The listing builds one solid part. Answer for the finished solid, in the listing's coordinates (mm). Face numbers are marked on the shaded views. A direction names the side the tool comes from. Round coordinates to 2 decimals unless told otherwise and drop trailing zeros. Write each loop counter-clockwise with the first axis right and the second up, starting at its lowest first coordinate (ties: lowest second). Pieces come first, ordered by that corner, then holes. Notation, with made-up numbers: M 42.5,87 L 99.5,87 A6 cw 99.5,92 Z; hole C 23,58.25 d10. An arc over 180 degrees is marked long. One line per item, written item: value. Start each with the question number.
(1) Consider probe 1 along X at (y, z) = (0, 6.5); probe 2 along X at (y, z) = (6, 10); probe 3 along Y at (x, z) = (0, 2.5). Determine where each line is inside the solid, lowest interval first.
(2) Section C-C (z = 5) is taken. Determine the outline of the cut face in (x, y).
(3) Section B-B (x = 0) is taken. Determine the outline of the cut face in (y, z).
(4) Given P1, Ø3, axis at x = 2, y = -16.5, coming from the +Z side; P2, Ø23, axis at x = 0, y = 0, coming from the +Z side, each flat-ended and moving along its own axis, determine where each tip first touches the part or whether it passes through.
(5) Section D-D (y = -15) is taken. Determine the outline of the cut face in (x, z), plus the area to 3 significant figures.
(6) Section A-A (y = 0) is taken. Determine the outline of the cut face in (x, z), plus the area to 3 significant figures.
(7) For a pull along X with two mould halves and no side action, classify the marked faces 1, 2, 3 and 4 as released by +X, released by -X, zero draft, split by the parting line, or undercut.
(8) For the marked faces 5, 6 and 7, determine the directions among +Z, -Z, +X, -X, +Y, -Y from which every point of the face is accessible in a straight line to the end or side of a thin tool.
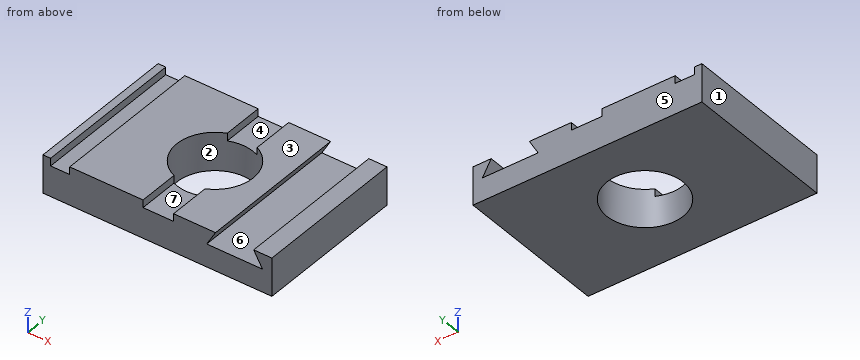
```python
from build123d import *

# Parameters (mm, degrees)
F0_W     = 76.2
F0_H     = 50.8
F0_R     = 12.7
F1_DEPTH = 12.7
F2_W     = 6.35
F2_H     = 50.8
F3_DEPTH = 2.54
F5_DEPTH = 50.801


with BuildPart() as f1:
    # F0 (on Top) → F1 (new body)
    with BuildSketch(Plane.XY):
        Rectangle(F0_W, F0_H)
        Circle(F0_R, mode=Mode.SUBTRACT)
    extrude(amount=F1_DEPTH)

    # F2 (on face) → F3 (cut)
    with BuildSketch(Plane.XY.offset(12.7)):
        with Locations((-32.385, 0)):
            Rectangle(F2_W, F2_H)
        with BuildLine():
            Line((5.37053629, 25.4), (-4.78946371, 25.4))
            Line((-4.78946371, 25.4), (-4.78946371, 11.7622717776))
            ThreePointArc((-4.78946371, 11.7622717776), (0.3170199067, 12.6960426267), (5.37053629, 11.5085767999))
            Line((5.37053629, 11.5085767999), (5.37053629, 25.4))
        make_face()
        with BuildLine():
            Line((-4.78946371, -11.7622717776), (-4.78946371, -25.4))
            Line((-4.78946371, -25.4), (5.37053629, -25.4))
            Line((5.37053629, -25.4), (5.37053629, -11.5085767999))
            ThreePointArc((5.37053629, -11.5085767999), (0.3170199067, -12.6960426267), (-4.78946371, -11.7622717776))
        make_face()
    extrude(amount=-F3_DEPTH, mode=Mode.SUBTRACT)

    # F4 (on face) → F5 (cut, through all)
    with BuildSketch(Plane.XZ.offset(25.4)):
        Polygon((32.04053629, 12.7), (19.34053629, 12.7), (16.4075969225, 7.62), (34.9734756574, 7.62), align=None)
    extrude(amount=-F5_DEPTH, mode=Mode.SUBTRACT)


solid = f1.part
```
Recorded:
1. probe 1: x = -38.1 to -12.7, 12.7 to 38.1
1. probe 2: x = -38.1 to -11.19, 11.19 to 17.78, 33.6 to 38.1
1. probe 3: y = -25.4 to -12.7, 12.7 to 25.4
2. outline: M -38.1,-25.4 L 38.1,-25.4 L 38.1,25.4 L -38.1,25.4 Z; hole C 0,0 d25.4
3. outline: M -25.4,0 L -12.7,0 L -12.7,10.16 L -25.4,10.16 Z; M 12.7,0 L 25.4,0 L 25.4,10.16 L 12.7,10.16 Z
4. P1: stops at z = 10.16
4. P2: passes through
5. outline: M -38.1,0 L 38.1,0 L 38.1,12.7 L 32.04,12.7 L 34.97,7.62 L 16.41,7.62 L 19.34,12.7 L 5.37,12.7 L 5.37,10.16 L -4.79,10.16 L -4.79,12.7 L -29.21,12.7 L -29.21,10.16 L -35.56,10.16 L -35.56,12.7 L -38.1,12.7 Z
5. area: 846 mm2
6. outline: M -38.1,0 L -12.7,0 L -12.7,12.7 L -29.21,12.7 L -29.21,10.16 L -35.56,10.16 L -35.56,12.7 L -38.1,12.7 Z; M 12.7,0 L 38.1,0 L 38.1,12.7 L 32.04,12.7 L 34.97,7.62 L 16.41,7.62 L 19.34,12.7 L 12.7,12.7 Z
6. area: 550 mm2
7. face 1: released by -X
7. face 2: undercut
7. face 3: zero draft
7. face 4: undercut
8. face 5: +Z, -Z, +X, -X, +Y
8. face 6: +Y, -Y
8. face 7: +Z, +Y, -Y
